```python
from build123d import *

# Parameters (mm, degrees)
F0_W     = 38.1
F0_H     = 25.4
F1_DEPTH = 6.35
F3_DEPTH = 6.35


with BuildPart() as f1:
    # F0 (on Top) → F1 (new body)
    with BuildSketch(Plane.XY):
        with Locations((19.05, 12.7)):
            Rectangle(F0_W, F0_H)
    extrude(amount=F1_DEPTH)

    # F2 (on Right) → F3 (join)
    with BuildSketch(Plane.YZ):
        with BuildLine():
            Line((0, 12.7), (0, 6.35))
            Line((0, 6.35), (25.4, 6.35))
            Line((25.4, 6.35), (25.4, 12.7))
            ThreePointArc((25.4, 12.7), (12.7, 25.4), (0, 12.7))
        make_face()
    extrude(amount=F3_DEPTH)


solid = f1.part
```
Source: CAD feature listing. Evaluate the final solid. Frame: model axes, mm. A direction names the side the tool comes from. Coordinates: 2 decimals unless noted, no trailing zeros. Write each loop counter-clockwise with the first axis right and the second up, starting at its lowest first coordinate (ties: lowest second). Pieces come first, ordered by that corner, then holes. Notation, with made-up numbers: M 43,47.25 L 97,47.25 A16 cw 97,67.25 Z; hole C 76.25,39 d1. An arc over 180 degrees is marked long. Answer as a JSON object with one key per item and string values.
1. Cut plane D-D on y = 18.25. Output: boundary loops of the cut face in (x, z).
Evaluation:
{"outline": "M 0,0 L 38.1,0 L 38.1,6.35 L 6.35,6.35 L 6.35,24.12 L 0,24.12 Z"}
2. Cut plane A-A on y = 12.7. Output: boundary loops of the cut face in (x, z).
Evaluation:
{"outline": "M 0,0 L 38.1,0 L 38.1,6.35 L 6.35,6.35 L 6.35,25.4 L 0,25.4 Z"}
3. Access query for faces 1 (the cylindrical face through (3.131, 12.979, 25.397)), 2 (the flat face through (22, 13, 6.35)). Directions: +Z, -Z, +X, -X, +Y, -Y. A direction counts if a zero-diameter tool reaches every point of the face in a straight line with its end or side. Return the directions, or none.
Evaluation:
{"face 1": "+Z, +X, -X", "face 2": "+Z, +X, +Y, -Y"}
4. Cut plane C-C on z = 8.25. Output: boundary loops of the cut face in (x, y).
Evaluation:
{"outline": "M 0,0 L 6.35,0 L 6.35,25.4 L 0,25.4 Z"}
5. Ray query, L1, parallel to Z at x = 17, y = 23.5; L2, parallel to Z at x = 3, y = 13. Return the intervals inside material, ascending.
Evaluation:
{"L1": "0 to 6.35", "L2": "0 to 25.4"}
6. Cut plane B-B on x = 16. Output: boundary loops of the cut face in (y, z), plus the area to 3 significant figures.
Evaluation:
{"outline": "M 0,0 L 25.4,0 L 25.4,6.35 L 0,6.35 Z", "area": "161 mm^2"}
7. Contact query for flat-ended pins moving along their axis: P1, Ø4, axis at x = 14.5, y = 15.5, coming from the +Z side; P2, Ø1.5, axis at y = 22.5, z = 15, coming from the +X side; P3, Ø5, axis at x = 25.5, z = 9, coming from the +Y side. Output: stop coordinate, or through.
Evaluation:
{"P1": "z = 6.35", "P2": "x = 6.35", "P3": "through"}
